from build123d import *

# Parameters (mm, degrees)
F0_W      = 168.275
F0_H      = 152.4
F1_DEPTH  = 44.45
F3_DEPTH  = 44.451
F4_W      = 23.8125
F4_H      = 19.05
F5_DEPTH  = 152.401
F7_DEPTH  = 19.05
F8_R      = 25.4
F9_DEPTH  = 63.501
F10_R     = 9.525
F11_DEPTH = 44.451
F12_R     = 15.875
F12_R_2   = 9.525
F13_DEPTH = 31.75


with BuildPart() as f1:
    # F0 (on Front) → F1 (new body)
    with BuildSketch(Plane.XZ):
        with Locations((-5.8413036168, -23.7527878196)):
            Rectangle(F0_W, F0_H)
    extrude(amount=F1_DEPTH)

    # F2 (on face) → F3 (cut, through all)
    with BuildSketch(Plane.XZ.offset(44.45)):
        Polygon((-89.9788036168, 52.4472121804), (-89.9788036168, -47.5652878196), (10.0336963832, 52.4472121804), align=None)
    extrude(amount=-F3_DEPTH, mode=Mode.SUBTRACT)

    # F4 (on face) → F5 (cut, through all)
    with BuildSketch(Plane(origin=(0, 0, -99.9527878196), x_dir=(1, 0, 0), z_dir=(0, 0, -1))):
        with Locations((-49.4975536168, 9.525)):
            Rectangle(F4_W, F4_H)
    extrude(amount=-F5_DEPTH, mode=Mode.SUBTRACT)

    # F6 (on face) → F7 (join)
    with BuildSketch(Plane.XZ.offset(44.45)):
        Polygon((-1.0788036168, -49.1527878196), (78.2961963832, -49.1527878196), (78.2961963832, 52.4472121804), (10.0336963832, 52.4472121804), (-16.9538036168, 25.4597121804), (-16.9538036168, -33.2777878196), align=None)
    extrude(amount=F7_DEPTH)

    # F8 (on face) → F9 (cut, through all)
    with BuildSketch(Plane.XZ.offset(63.5)):
        with Locations((33.8461963832, 7.9972121804)):
            Circle(F8_R)
        Polygon((78.2961963832, 52.4472121804), (62.4211963832, 52.4472121804), (78.2961963832, 36.5722121804), align=None)
    extrude(amount=-F9_DEPTH, mode=Mode.SUBTRACT)

    # F10 (on face) → F11 (cut, through all)
    with BuildSketch(Plane.XZ.offset(44.45)):
        with Locations((33.8461963832, -74.5527878196)):
            Circle(F10_R)
    extrude(amount=-F11_DEPTH, mode=Mode.SUBTRACT)

    # F12 (on face) → F13 (cut)
    with BuildSketch(Plane(origin=(0, 0, 0), x_dir=(-1, 0, 0), z_dir=(0, 1, 0))):
        with Locations((-33.8461963832, -74.5527878196)):
            Circle(F12_R)
        with Locations((-33.8461963832, -74.5527878196)):
            Circle(F12_R_2, mode=Mode.SUBTRACT)
    extrude(amount=-F13_DEPTH, mode=Mode.SUBTRACT)


solid = f1.part
CAD build for the part. Positions are in the model's coordinates, mm. A direction names the side the tool comes from. Round coordinates to 2 decimals unless told otherwise and drop trailing zeros. Write each loop counter-clockwise with the first axis right and the second up, starting at its lowest first coordinate (ties: lowest second). Pieces come first, ordered by that corner, then holes. Notation, with made-up numbers: (3, -37.5) -> (10, -37.5) arc R12 cw to (10, -24.5) -> close; hole circle Ø11 at (-15, -7.5). An arc over 180 degrees is marked (long way). Answer as a JSON object with one key per item and string values.
(1) Band-saw the part on B-B, the plane x = 54.5. List the corners of the cut face in (y, z), then the cut area to 3 significant figures.
Reported:
{"outline": "(-63.5, -49.15) -> (-44.45, -49.15) -> (-44.45, -99.95) -> (0, -99.95) -> (0, -6.79) -> (-63.5, -6.79) -> close; (-63.5, 22.78) -> (0, 22.78) -> (0, 52.45) -> (-63.5, 52.45) -> close", "area": "6,830 mm^2"}
(2) Band-saw the part on C-C, the plane z = 11.5. List the corners of the cut face in (x, y), then the cut area to 3 significant figures.
Reported:
{"outline": "(-30.91, -44.45) -> (-16.95, -44.45) -> (-16.95, -63.5) -> (8.69, -63.5) -> (8.69, 0) -> (-30.91, 0) -> close; (59, -63.5) -> (78.3, -63.5) -> (78.3, 0) -> (59, 0) -> close", "area": "3,470 mm^2"}
(3) Probe probe 1 along X at (y, z) = (-15.5, -61); probe 2 along Y at (x, z) = (-22, -19.5); probe 3 along Z at (x, y) = (21, -18). List the from-to ranges inside material, lowest first. Write a range as [from, to].
Reported:
{"probe 1": "x = [-89.98, -61.4], [-37.59, 25.58], [42.11, 78.3]", "probe 2": "y = [-44.45, 0]", "probe 3": "z = [-99.95, -83.88], [-65.23, -13.91], [29.91, 52.45]"}
(4) Two-plate mould, pull along Z, no slides. Class faces 1 (the face through (-37.591, -9, -48)), 2 (the face through (70.25, -32.19, 44.62)), 3 (the face through (38.967, -38.189, -66.521)): +Z half, -Z half, draft (parallel to the pull), parting line (faces both ways), or undercut.
Reported:
{"face 1": "draft", "face 2": "+Z half", "face 3": "undercut"}
(5) Pin check, flat tips, straight feed: P1, Ø7, axis at x = -54.5, z = -38.5, coming from the +Y side; P2, Ø8, axis at x = -24.5, y = -33.5, coming from the +Z side; P3, Ø5.5, axis at y = -53.5, z = 5, coming from the -X side. Stop position of each tip, or through.
Reported:
{"P1": "stops at y = -19.05", "P2": "stops at z = 21.91", "P3": "stops at x = -16.95"}
(6) Band-saw the part on D-D, the plane x = 30. List the corners of the cut face in (y, z).
Reported:
{"outline": "(-63.5, -49.15) -> (-44.45, -49.15) -> (-44.45, -65.84) -> (-31.75, -65.84) -> (-31.75, -59.15) -> (0, -59.15) -> (0, -17.11) -> (-63.5, -17.11) -> close; (-63.5, 33.1) -> (0, 33.1) -> (0, 52.45) -> (-63.5, 52.45) -> close; (-44.45, -99.95) -> (0, -99.95) -> (0, -89.95) -> (-31.75, -89.95) -> (-31.75, -83.27) -> (-44.45, -83.27) -> close"}
(7) Band-saw the part on A-A, the plane y = -15. List the corners of the cut face in (x, z) (3 decimals), then the cut area to 3 significant figures.
Reported:
{"outline": "(-89.979, -99.953) -> (-61.404, -99.953) -> (-61.404, -18.99) -> (-89.979, -47.565) -> close; (-37.591, -99.953) -> (78.296, -99.953) -> (78.296, 36.572) -> (62.421, 52.447) -> (10.034, 52.447) -> (-37.591, 4.822) -> close; hole circle Ø50.8 at (33.846, 7.997); hole circle Ø31.75 at (33.846, -74.553)", "area": "15,500 mm^2"}
(8) Which spindle directions (+Z, -Z, +X, -X, +Y, -Y) get a long thin tool onto all of the face, cutting with end or side? Do faces 4 (the face through (-7, -44.45, -64)), 5 (the face through (27, -31.75, -81.4)), 6 (the face through (-61.404, -9, -60)), 7 (the face through (-16.954, -54, -3)). Say none if no direction does.
Reported:
{"face 4": "-Z, -X, -Y", "face 5": "+Y", "face 6": "+Z, -Z, +Y", "face 7": "+Z, -Z, -X, -Y"}
